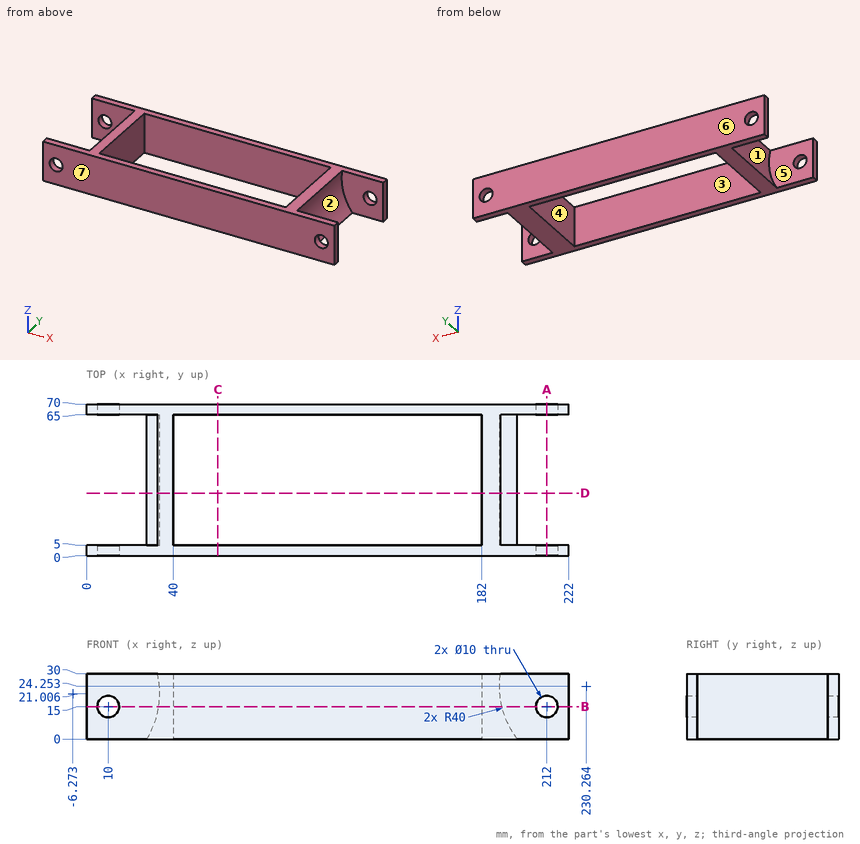
Input: dimensioned drawing with shaded views. Units: mm. Origin: part minimum x, y, z. A direction names the side the tool comes from. Coordinates: 2 decimals unless noted, no trailing zeros. Order: outer loops, then holes, each group sorted by start corner. A loop starts at its lowest first (then second) coordinate and runs counter-clockwise, first axis right, second up. Notation, with made-up numbers: (32.25, -24.75) - (63.25, -24.75) arc R24 cw to (63.25, -10.75) - close; hole circle Ø6 at (21.25, 10.5). An arc over 180 degrees is marked (long way). Put each result on its own line as item: value.
1. Cut plane C-C on x = 60.5. Return the cut outline in (y, z), then the cut area to 3 significant figures.
Report:
outline: (0, 0) - (5, 0) - (5, 30) - (0, 30) - close; (65, 0) - (70, 0) - (70, 30) - (65, 30) - close
area: 300 mm2
2. Cut plane D-D on y = 29. Return the cut outline in (x, z) (1 decimal).
Report:
outline: (27.8, 0) - (40, 0) - (40, 30) - (32.7, 30) arc R40 cw to start; (182, 0) - (198.5, 0) arc R40 cw to (190.7, 30) - (182, 30) - close
3. Cut plane A-A on x = 212. Return the cut outline in (y, z).
Report:
outline: (0, 0) - (5, 0) - (5, 10) - (0, 10) - close; (0, 20) - (5, 20) - (5, 30) - (0, 30) - close; (65, 0) - (70, 0) - (70, 10) - (65, 10) - close; (65, 20) - (70, 20) - (70, 30) - (65, 30) - close
4. Line query: line 1 along X through (y, z) = (67.8, 15); line 2 along Y through (x, z) = (144.5, 4.5); line 3 along Z through (x, y) = (212, 67). Output: solid intervals per line, ascending.
Report:
line 1: x = 0 to 5, 15 to 207, 217 to 222
line 2: y = 0 to 5, 65 to 70
line 3: z = 0 to 10, 20 to 30
5. Draft query along Y for the marked faces 4, 5, 6 and 7. Return one class per face: pulls with the +Y half, pulls with the -Y half, needs draft (parallel to the pull), parting line crosses it, or undercut.
Report:
face 4: undercut
face 5: undercut
face 6: pulls with the +Y half
face 7: pulls with the -Y half
6. Reachability of the marked faces 1, 2 and 3 from +Z, -Z, +X, -X, +Y, -Y: full face, straight path, thin tool, end or side. Return the list, or none.
Report:
face 1: -X
face 2: +X
face 3: +Z, -Z
7. Cut plane B-B on z = 15. State how many separate pieces and enclosed holes the cut face has.
Report:
separate pieces: 5
enclosed holes: 1
8. Contact query for flat-ended pins moving along their axis: pin 1 Ø8 at (x, z) = (212, 15) entering from +Y; pin 2 Ø1 at (y, z) = (16.5, 24.5) entering from -X; pin 3 Ø9 at (y, z) = (25, 17) entering from +X; pin 4 Ø10 at (y, z) = (48, 25.5) entering from -X. Output: stop coordinate, or through.
Report:
pin 1: passes through
pin 2: stops at x = 33.53
pin 3: stops at x = 192.03
pin 4: stops at x = 32.7
